Autodesk Fusion 360 part; units mm, degrees
sketch "Sketch1" plane through (0, 0, 0) normal (0, 0, 1) x (1, 0, 0)
  line L0 (-7.5, 14.2587) -> (-2.5, 14.2587)
  line L1 (-2.0653, 12.85) -> (-2.0653, 5.5267)
  arc A0 (-7.8282, 5.1403) -> (7.8282, 5.1403) centre (0, 0) ccw
  line L2 (-1.565, 12.3091) -> (-1.565, 5.6887)
  line L3 (-2.0653, 5.5267) -> (-2.0653, 12.85)
  line L4 (-7.5, 14.2587) -> (-2.5, 14.2587)
  line L5 (2.5, 14.2587) -> (7.5, 14.2587)
  arc A1 (-2.0653, 5.5267) -> (-1.565, 5.6887) centre (0, 0) ccw
  line L6 (-2.5, -19.9263) -> (2.5, -19.9263)
  arc A2 (-1.565, 12.3091) -> (2.5, 14.2587) centre (0, 14.2587) ccw
  arc A3 (-2.5, 14.2587) -> (-2.0653, 12.85) centre (0, 14.2587) ccw
  line L7 (0, 0) -> (-7.5, 0)
  line L8 (-7.5, 6.238) -> (-7.5, 14.2587)
  line L9 (0, 0) -> (7.5, 0)
  line L10 (7.5, 6.238) -> (7.5, 14.2587)
  line L11 (0, 17.4341) -> (0, 17.3504)
  arc A4 (-7.8282, 5.1403) -> (-7.5, 6.238) centre (-9.5, 6.238) ccw
  arc A5 (7.5, 6.238) -> (7.8282, 5.1403) centre (9.5, 6.238) ccw
  dimension "d1" = 11.8
  dimension "d5" = 5
  dimension "d25" = 7.5
  dimension "d26" = 7.5
  dimension "d27" = 2
extrude "Extrude1" add sketch "Sketch1" along normal blind 6 contours L0 L1 A0 L2 L3 L4 L5 A1 A2 A3 L8 L10 A4 A5
hole "Hole1" at (-7.5, 7.2587, 3) direction (1, 0, 0) diameter 2.4 depth 5.6892 tip angle 180
hole "Hole2" at (-1.565, 7.2768, 3) direction (1, 0, 0) diameter 1.5 depth 8.4147 tip angle 180
sketch "Sketch2" plane through (0, 14.2587, 0) normal (0, 1, 0) x (-1, 0, 0)
  line L0 (7.5233, 0) -> (-7.4993, 0)
  line L1 (-7.4993, 0) -> (-7.4993, 6.0044)
  line L2 (-7.4993, 6.0044) -> (7.5233, 6.0044)
  line L3 (7.5233, 6.0044) -> (7.5233, 0)
  line L4 (7.5233, 3.0022) -> (-7.4993, 3.0022)
  line L5 (6.012, 2.0757) -> (-5.988, 2.0757)
  line L6 (-5.988, 2.0757) -> (-5.988, 3.9288)
  line L7 (-5.988, 3.9288) -> (6.012, 3.9288)
  line L8 (6.012, 3.9288) -> (6.012, 2.0757)
  line L9 (6.012, 2.0757) -> (-5.988, 3.9288) construction
  line L10 (-5.988, 2.0757) -> (6.012, 3.9288) construction
  point P0 (0.012, 3.0022)
  dimension "d30" = 12
hole "Hole3" at (5.991, 14.2587, 3.0012) direction (0, -1, 0) diameter 1.5 depth 5 tip angle 180
hole "Hole4" at (-6.0143, 14.2587, 3.0029) direction (0, -1, 0) diameter 1.5 depth 5 tip angle 180
The model under review builds one solid part; all positions refer to its coordinate system, in mm. A direction names the side the tool comes from. Give positions to 0.01 mm unless a question says otherwise; leave off trailing zeros. Write each loop counter-clockwise with the first axis right and the second up, starting at its lowest first coordinate (ties: lowest second). Pieces come first, ordered by that corner, then holes. Notation, with made-up numbers: M 63.5,3 L 83.5,3 A19 cw 83.5,25 Z; hole C 31.5,65 d7. An arc over 180 degrees is marked long. Write item = value, one per line. Start each with the question number.
Q1. We need section C-C (z = 3). State the section outline as (x, y) points (3 decimals), plus the area to 3 significant figures.
Q2. We need section D-D (y = 13.25). State the section outline as (x, z) points, plus the area to 3 significant figures.
Q3. Clearance check with flat-ended pins moving along their axes: pin 1 (1 mm diameter, centred on x = -3, z = 3, fed in from -Y); pin 2 (4 mm diameter, centred on x = 7, y = -6.5, fed in from +Z); pin 3 (1.8 mm diameter, centred on y = 11, z = 3.5, fed in from +X); pin 4 (1 mm diameter, centred on x = 2.5, z = 5, fed in from -Y). State where each tip first meets the part, or that it passes through.
Q4. Mouldability with a two-part tool opening along X and no side actions: class faces 4 (the face through (-1.565, 9, 3)), 5 (the face through (7.5, 10, 3)), 6 (the face through (5, 14.259, 3)) as released by +X, released by -X, zero draft, split by the parting line, or undercut.
Q5. We need section B-B (y = 0). State the section outline as (x, z) points (3 decimals), plus the area to 3 significant figures.
Q6. Machinability: for faces 1 (the face through (-2.065, 9, 3)), 2 (the face through (-7.5, 10, 3)), 3 (the face through (6, 9.259, 3)), which of the approach directions +Z, -Z, +X, -X, +Y, -Y give a long, thin tool a straight path to every point of the face, cutting with its end or side? Answer none if there is none.
Q7. For line 1 (X direction, y = 8, z = 0.95) (3 decimals); line 2 (Y direction, x = -5.25, z = 2.4); line 3 (X direction, y = 0, z = 1) (3 decimals), list the stretches that pass through material, from the lowest coordinate up.
Q8. We need section A-A (x = 2). State the section outline as (y, z) points, plus the area to 3 significant figures.
Result set:
q1.outline = M -7.828,5.14 A9.365 ccw long 7.828,5.14 A2 cw 7.5,6.238 L 7.5,14.259 L 6.741,14.259 L 6.741,9.259 L 5.241,9.259 L 5.241,14.259 L 2.5,14.259 A2.5 cw -1.565,12.309 L -1.565,8.027 L 6.85,8.027 L 6.85,6.527 L -1.565,6.527 L -1.565,5.689 A5.9 cw long -2.065,5.527 L -2.065,6.059 L -7.5,6.059 L -7.5,6.238 A2 cw Z; M -7.5,8.459 L -2.065,8.459 L -2.065,12.85 A2.5 cw -2.5,14.259 L -5.264,14.259 L -5.264,9.259 L -6.764,9.259 L -6.764,14.259 L -7.5,14.259 Z
q1.area = 203 mm2
q2.outline = M -7.5,0 L -2.29,0 L -2.29,6 L -7.5,6 Z; M 2.29,0 L 7.5,0 L 7.5,6 L 2.29,6 Z; hole C -6.01,3 d1.5; hole C 5.99,3 d1.5
q2.area = 59.0 mm2
q3.pin_1 = -9.03
q3.pin_2 = 6
q3.pin_3 = 7.5
q3.pin_4 = -9.15
q4.face_4 = undercut
q4.face_5 = released by +X
q4.face_6 = zero draft
q5.outline = M -9.365,0 L -5.899,0 L -5.899,6 L -9.365,6 Z; M 5.901,0 L 9.365,0 L 9.365,6 L 5.901,6 Z
q5.area = 41.6 mm2
q6.face_1 = +Z, -Z, +Y
q6.face_2 = +Z, -Z, -X, +Y
q6.face_3 = +Y
q7.line_1 = -7.5 to -2.065, -1.565 to 7.5
q7.line_2 = -7.76 to -2.69, 2.69 to 6.22, 8.3 to 14.26
q7.line_3 = -9.365 to -5.899, 5.901 to 9.365
q8.outline = M -9.15,0 L -5.55,0 L -5.55,6 L -9.15,6 Z; M 5.55,0 L 12.76,0 L 12.76,6 L 5.55,6 Z; hole C 7.28,3 d1.5
q8.area = 63.1 mm2
